For this review, take the finished solid that the model builds, in its own axes (mm). A direction names the side the tool comes from. Round coordinates to 2 decimals unless told otherwise and drop trailing zeros. Write each loop counter-clockwise with the first axis right and the second up, starting at its lowest first coordinate (ties: lowest second). Pieces come first, ordered by that corner, then holes. Notation, with made-up numbers: M 9,60.5 L 64,60.5 A29 cw 64,97.5 Z; hole C 80.25,-9 d3. An arc over 180 degrees is marked long. Answer in a Markdown table with one row per item.
```python
from build123d import *

# Parameters (mm, degrees)
BOSS_EXTRUDE1_DEPTH = 15
SKETCH2_W           = 19.139819484
SKETCH2_H           = 3.3
CUT_EXTRUDE1_DEPTH  = 3
CHAMFER1_SIZE       = 3
BOSS_EXTRUDE2_DEPTH = 2
CUT_EXTRUDE2_DEPTH  = 15
CUT_EXTRUDE3_DEPTH  = 8.5


with BuildPart() as part:
    # Sketch1 → Boss-Extrude1 (new body)
    with BuildSketch(Plane(origin=(0, 0, 0), x_dir=(1, 0, 0), z_dir=(0, 1, 0))):
        Polygon((-5, 8.5), (10, 8.5), (10, 23.5), (23.5, 23.5), (23.5, -5), (-5, -5), align=None)
        Polygon((0, 0), (0, 3.5), (15, 3.5), (15, 18.5), (18.5, 18.5), (18.5, 0), align=None, mode=Mode.SUBTRACT)
    extrude(amount=BOSS_EXTRUDE1_DEPTH)

    # Sketch2 → Cut-Extrude1 (cut)
    with BuildSketch(Plane(origin=(0, 0, -8.5), x_dir=(-1, 0, 0), z_dir=(0, 0, -1))):
        with Locations((-0.430090258, 8.5)):
            Rectangle(SKETCH2_W, SKETCH2_H)
    extrude(amount=-CUT_EXTRUDE1_DEPTH, mode=Mode.SUBTRACT)

    # Chamfer1
    chamfer1_edges = [part.edges().sort_by_distance(p)[0] for p in [
        (2.5, 6.85, -8.5),
        (2.5, 10.15, -8.5),
    ]]
    chamfer(chamfer1_edges, length=CHAMFER1_SIZE - 0.0001)  # a hair under: the kernel refuses the full size

    # Sketch4 → Boss-Extrude2 (add)
    with BuildSketch(Plane(origin=(0, 15, 0), x_dir=(1, 0, 0), z_dir=(0, 1, 0))):
        Polygon((-5, 8.5), (10, 8.5), (10, 23.5), (23.5, 23.5), (23.5, -5), (-5, -5), align=None)
    extrude(amount=BOSS_EXTRUDE2_DEPTH)

    # Sketch5 → Cut-Extrude2 (cut)
    with BuildSketch(Plane.XZ):
        Polygon((0, 0), (-5, 0), (-5, -3.5), (15, -3.5), (15, -24.324803995), (18.5, -24.324803995), (18.5, 0), align=None)
    extrude(amount=-CUT_EXTRUDE2_DEPTH, mode=Mode.SUBTRACT)

    # Sketch6 → Cut-Extrude3 (cut)
    with BuildSketch(Plane.ZY.offset(-10)):
        Polygon((-5.5, 10.15), (-5.5, 6.85), (-8.5, 3.85), (-8.5, 0), (-23.5, 0), (-23.5, 10.15), align=None)
    extrude(amount=-CUT_EXTRUDE3_DEPTH, mode=Mode.SUBTRACT)


solid = part.part
```
Q1. Take a section at D-D (x = 16.25). State the section outline as (y, z) points.
Found:
| item | result |
|---|---|
| outline | M 0,0 L 15,0 L 15,-23.5 L 17,-23.5 L 17,5 L 0,5 Z |
Q2. Take a section at A-A (y = 13.5). State the section outline as (x, z) points, then the cut area to 3 significant figures.
Found:
| item | result |
|---|---|
| outline | M -5,-8.5 L 10,-8.5 L 10,-23.5 L 15,-23.5 L 15,-3.5 L -5,-3.5 Z; M -5,0 L 18.5,0 L 18.5,-23.5 L 23.5,-23.5 L 23.5,5 L -5,5 Z |
| area | 435 mm² |
Q3. Mouldability with a two-part tool opening along Y and no side actions: class faces 5 (the face through (13, 17, -6)), 6 (the face through (2.6, 11.63, -6.98)), 7 (the face through (5, 2, -8.5)) as +Y half, -Y half, draft (parallel to the pull), parting line (faces both ways), or undercut.
Found:
| item | result |
|---|---|
| face 5 | +Y half |
| face 6 | undercut |
| face 7 | draft |
Q4. Take a section at B-B (z = -4.75). State the section outline as (x, y) points.
Found:
| item | result |
|---|---|
| outline | M -5,0 L 15,0 L 15,15 L 18.5,15 L 18.5,0 L 23.5,0 L 23.5,17 L -5,17 Z |
Q5. Machinability: for faces 1 (the face through (15, 11, -11)), 2 (the face through (5, 9, -5.5)), 3 (the face through (5, 7, -3.5)), 4 (the face through (2, 15, -8.5)), which of the approach directions +Z, -Z, +X, -X, +Y, -Y give a long, thin tool a straight path to every point of the face, cutting with its end or side? Answer none if there is none.
Found:
| item | result |
|---|---|
| face 1 | -Z, -Y |
| face 2 | -Z, -X |
| face 3 | -X, -Y |
| face 4 | -Z, -X, +Y, -Y |
Q6. Insertion check: P1, Ø1.9, axis at x = 1, y = 14.5, coming from the -Z side; P2, Ø8, axis at y = 5.5, z = -13, coming from the -X side; P3, Ø5, axis at y = 9.5, z = -12.5, coming from the -X side. Each pin has a flat end and moves straight along its axis. Give the tip position at first contact, or say it passes through.
Found:
| item | result |
|---|---|
| P1 | z = -8.5 |
| P2 | x = 18.5 |
| P3 | x = 10 |
Q7. Take a section at C-C (y = 15.5). State the section outline as (x, z) points.
Found:
| item | result |
|---|---|
| outline | M -5,-8.5 L 10,-8.5 L 10,-23.5 L 23.5,-23.5 L 23.5,5 L -5,5 Z |
Q8. For probe 1 along X at (y, z) = (14.5, -20); probe 2 along Z at (x, y) = (8.75, 9.5); probe 3 along Z at (x, y) = (13.25, 1), list the stretches that pass through material, from the lowest coordinate up.
Found:
| item | result |
|---|---|
| probe 1 | 10 to 15, 18.5 to 23.5 |
| probe 2 | -5.5 to -3.5, 0 to 5 |
| probe 3 | -8.5 to -3.5, 0 to 5 |
